Could you check a few things on this drawing? It's one solid part, dimensions in mm from its lowest x, y, z. Give positions to 0.01 mm unless a question says otherwise; leave off trailing zeros. Loops run counter-clockwise (first coordinate to the right, second up) from the corner with the lowest first, then second, coordinate; pieces in that order, holes last. Notation, with made-up numbers: M 5.25,62.5 L 18.25,62.5 A24 ccw 18.25,90.5 Z; hole C 17.5,79.25 d8. An arc over 180 degrees is marked long. Return JSON: item names as keys, results as strings. Group by question number.
1. Please list where these lines run through material, in increasing order: line 1 (X direction, y = 8.25, z = 24.5); line 2 (Z direction, x = 17, y = 12).
2. If we section it at C-C (y = 8.5): State how many separate pieces and enclosed holes the cut face has, plus the area to 3 significant figures.
3. If we mould it in two halves opening along X, with no side actions, what happens to the marked faces 1, 2 and 3? For each: +X half, -X half, draft (parallel to the pull), parting line (faces both ways), or undercut.
4. If we section it at A-A (z = 24.5): Write out the boundary of the cut face in (x, y).
5. If we section it at B-B (x = 24.5): Write out the boundary of the cut face in (y, z).
6. For pin 1 (6 mm diameter, centred on y = 10.5, z = 15.5, fed in from -X); pin 2 (1.5 mm diameter, centred on x = 13, y = 8, fed in from +Z); pin 3 (6 mm diameter, centred on x = 18, y = 11.5, fed in from -Z); pin 4 (5 mm diameter, centred on x = 16.75, z = 32.25, fed in from -Y), each with a flat end and sliding along its axis, tell me the tip position at first contact or that it passes through.
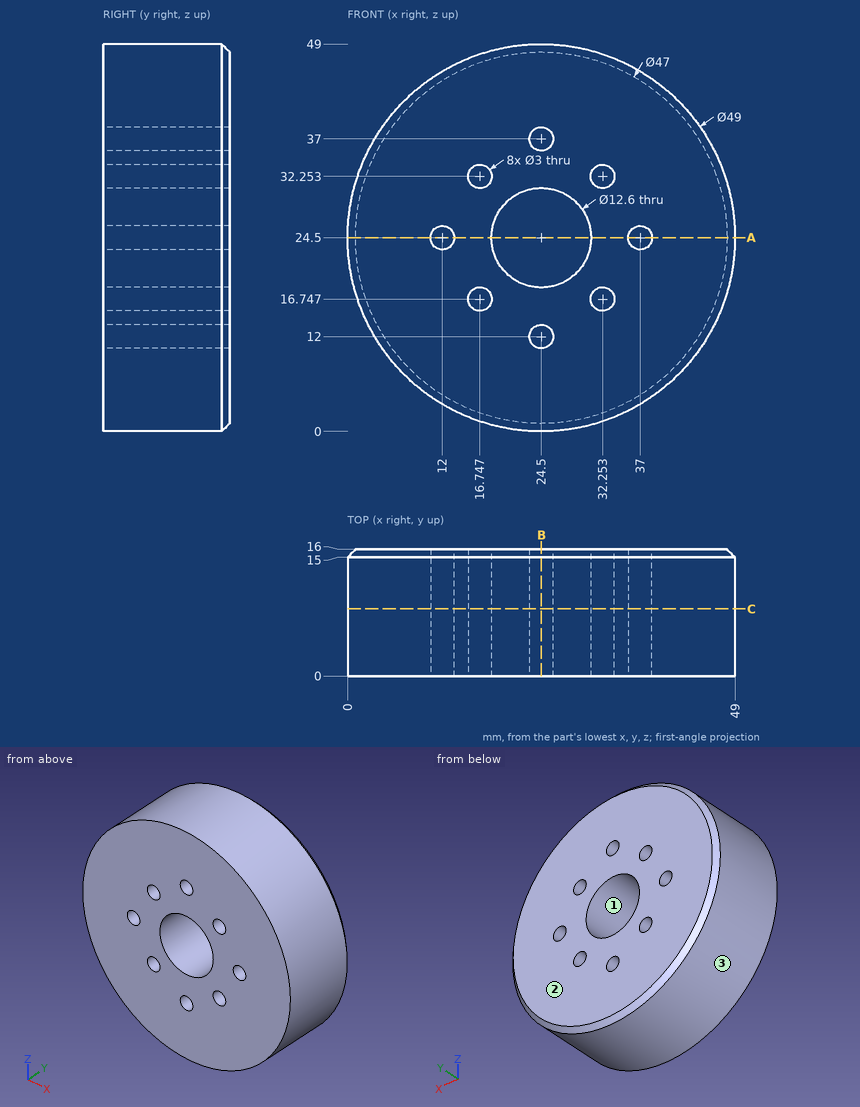
Answer:
{
 "1": {"line 1": "x = 0 to 10.5, 13.5 to 18.2, 30.8 to 35.5, 38.5 to 49", "line 2": "z = 1.18 to 15.27, 18.23 to 30.77, 33.73 to 47.82"},
 "2": {"separate pieces": "1", "enclosed holes": "9", "area": "1,700 mm²"},
 "3": {"face 1": "undercut", "face 2": "draft", "face 3": "parting line"},
 "4": {"outline": "M 0,0 L 10.5,0 L 10.5,16 L 1,16 L 0,15 Z; M 13.5,0 L 18.2,0 L 18.2,16 L 13.5,16 Z; M 30.8,0 L 35.5,0 L 35.5,16 L 30.8,16 Z; M 38.5,0 L 49,0 L 49,15 L 48,16 L 38.5,16 Z"},
 "5": {"outline": "M 0,0 L 15,0 L 16,1 L 16,10.5 L 0,10.5 Z; M 0,13.5 L 16,13.5 L 16,18.2 L 0,18.2 Z; M 0,30.8 L 16,30.8 L 16,35.5 L 0,35.5 Z; M 0,38.5 L 16,38.5 L 16,48 L 15,49 L 0,49 Z"},
 "6": {"pin 1": "stops at x = 0.75", "pin 2": "stops at z = 46.52", "pin 3": "stops at z = 0.25", "pin 4": "stops at y = 0"}
}
